For this review, take the finished solid that the model builds, in its own axes (mm). Round coordinates to 2 decimals unless told otherwise and drop trailing zeros. Order: outer loops, then holes, each group sorted by start corner. A loop starts at its lowest first (then second) coordinate and runs counter-clockwise, first axis right, second up. Notation, with made-up numbers: (86, 61) - (123, 61) arc R17 cw to (123, 66) - close; hole circle Ø10 at (-5, -9). An arc over 180 degrees is marked (long way). Write each question's results on one line, items separated by ' | '. Start each with the question number.
(1) Insertion check: pin 1 Ø1.2 at (y, z) = (3, 12) entering from -X. The pin has a flat end and moves straight along its axis. Give the tip position at first contact, or say it passes through.
(2) Take a section at B-B, the plane y = 2.6. Give the boundary of the cut face in (x, z).
(3) Take a section at C-C, the plane z = 4.5. Give the boundary of the cut face in (x, y).
(4) For L1, parallel to Z at x = -19, y = 2.75; L2, parallel to Z at x = 12, y = 1.65; L3, parallel to X at y = 1.4, z = -49.25, list the stretches that pass through material, from the lowest coordinate up. Write a range as from..to.
(5) Take a section at A-A, the plane x = -13. Give the boundary of the cut face in (y, z), plus the area to 3 significant figures.
(6) Take a section at D-D, the plane z = 40.5. Give the boundary of the cut face in (x, y), plus the area to 3 significant figures.
```python
from build123d import *

# Parameters (mm, degrees)
SKETCH1_R           = 1.6
BOSS_EXTRUDE1_DEPTH = 4


with BuildPart() as part:
    # Sketch1 → Boss-Extrude1 (new body)
    # profile 1 of 5: a face of its own
    with BuildSketch(Plane(origin=(0, 0, 0), x_dir=(1, 0, 0), z_dir=(0, 1, 0))):
        with BuildLine():
            Line((-20, 44.25), (0, 44.25))
            ThreePointArc((0, 44.25), (5, 49.25), (0, 54.25))
            Line((0, 54.25), (-20, 54.25))
            ThreePointArc((-20, 54.25), (-25, 49.25), (-20, 44.25))
        make_face()
        with Locations(Location((0, 49.25, 0), (0, 0, 270))):
            Circle(SKETCH1_R, mode=Mode.SUBTRACT)
        with Locations(Location((-20, 49.25, 0), (0, 0, 270))):
            Circle(SKETCH1_R, mode=Mode.SUBTRACT)
    # profile 2 of 5: a face of its own
    with BuildSketch(Plane(origin=(0, 0, 0), x_dir=(1, 0, 0), z_dir=(0, 1, 0))):
        with BuildLine():
            Line((13.735803892, 49.084798783), (1.875803892, 53.884798783))
            ThreePointArc((1.875803892, 53.884798783), (4.907850544, 48.294488073), (0, 44.25))
            ThreePointArc((0, 44.25), (4.850752519, 42.240752519), (6.86, 37.39))
            Line((6.86, 37.39), (6.86, 44.45))
            ThreePointArc((6.86, 44.45), (9.065274563, 48.596023363), (13.735803892, 49.084798783))
        make_face()
    # profile 3 of 5: a face of its own
    with BuildSketch(Plane(origin=(0, 0, 0), x_dir=(1, 0, 0), z_dir=(0, 1, 0))):
        with BuildLine():
            ThreePointArc((6.86, -44.45), (11.86, -49.45), (16.86, -44.45))
            Line((16.86, -44.45), (16.86, 44.45))
            ThreePointArc((16.86, 44.45), (11.86, 49.45), (6.86, 44.45))
            Line((6.86, 44.45), (6.86, -44.45))
        make_face()
        with Locations(Location((11.86, -44.45, 0), (0, 0, 270))):
            Circle(SKETCH1_R, mode=Mode.SUBTRACT)
        with Locations(Location((11.86, 44.45, 0), (0, 0, 270))):
            Circle(SKETCH1_R, mode=Mode.SUBTRACT)
    # profile 4 of 5: a face of its own
    with BuildSketch(Plane(origin=(0, 0, 0), x_dir=(1, 0, 0), z_dir=(0, 1, 0))):
        with BuildLine():
            ThreePointArc((0, -44.25), (5, -49.25), (0, -54.25))
            Line((0, -54.25), (-20, -54.25))
            ThreePointArc((-20, -54.25), (-25, -49.25), (-20, -44.25))
            Line((-20, -44.25), (0, -44.25))
        make_face()
        with Locations(Location((-20, -49.25, 0), (0, 0, 270))):
            Circle(SKETCH1_R, mode=Mode.SUBTRACT)
        with Locations(Location((0, -49.25, 0), (0, 0, 270))):
            Circle(SKETCH1_R, mode=Mode.SUBTRACT)
    # profile 5 of 5: a face of its own
    with BuildSketch(Plane(origin=(0, 0, 0), x_dir=(1, 0, 0), z_dir=(0, 1, 0))):
        with BuildLine():
            Line((6.86, -44.45), (6.86, -37.39))
            ThreePointArc((6.86, -37.39), (4.850752519, -42.240752519), (0, -44.25))
            ThreePointArc((0, -44.25), (4.907850544, -48.294488073), (1.875803892, -53.884798783))
            Line((1.875803892, -53.884798783), (13.735803892, -49.084798783))
            ThreePointArc((13.735803892, -49.084798783), (9.065274563, -48.596023363), (6.86, -44.45))
        make_face()
    extrude(amount=BOSS_EXTRUDE1_DEPTH)


solid = part.part
```
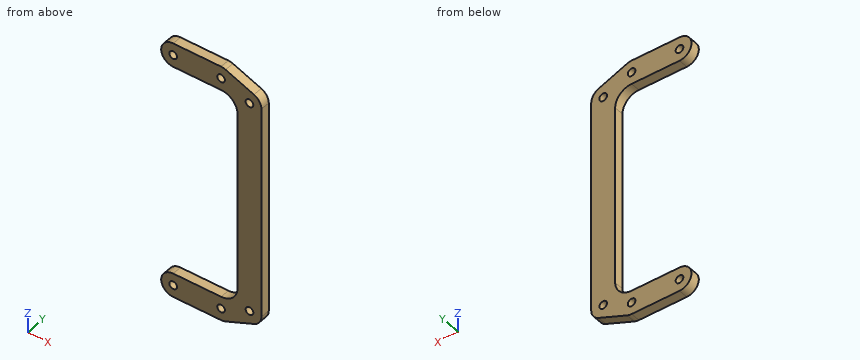
Results below:
1) pin 1: stops at x = 6.86
2) outline: (-20, -54.25) - (0, -54.25) arc R5 ccw to (1.88, -53.88) - (13.74, -49.08) arc R5 ccw to (16.86, -44.45) - (16.86, 44.45) arc R5 ccw to (13.74, 49.08) - (1.88, 53.88) arc R5 ccw to (0, 54.25) - (-20, 54.25) arc R5 ccw to (-20, 44.25) - (0, 44.25) arc R6.86 cw to (6.86, 37.39) - (6.86, -37.39) arc R6.86 cw to (0, -44.25) - (-20, -44.25) arc R5 ccw to start; hole circle Ø3.2 at (-20, -49.25); hole circle Ø3.2 at (-20, 49.25); hole circle Ø3.2 at (0, -49.25); hole circle Ø3.2 at (0, 49.25); hole circle Ø3.2 at (11.86, -44.45); hole circle Ø3.2 at (11.86, 44.45)
3) outline: (6.86, 0) - (16.86, 0) - (16.86, 4) - (6.86, 4) - close
4) L1: z = -54.25..-50.5, -48..-44.25, 44.25..48, 50.5..54.25 | L2: z = -49.79..-46.04, -42.86..42.86, 46.04..49.79 | L3: x = -25..-21.6, -18.4..-1.6, 1.6..13.33
5) outline: (0, -54.25) - (4, -54.25) - (4, -44.25) - (0, -44.25) - close; (0, 44.25) - (4, 44.25) - (4, 54.25) - (0, 54.25) - close | area: 80.0 mm^2
6) outline: (6.11, 0) - (16.86, 0) - (16.86, 4) - (6.11, 4) - close | area: 43.0 mm^2
